from build123d import *

# Parameters (mm, degrees)
SKETCH1_W           = 4.1
SKETCH1_H           = 15
SKETCH1_W_2         = 15
SKETCH1_H_2         = 4.1
BOSS_EXTRUDE1_DEPTH = 4.1


with BuildPart() as part:
    # Sketch1 → Boss-Extrude1 (new body)
    with BuildSketch(Plane(origin=(0, 0, 0), x_dir=(1, 0, 0), z_dir=(0, 1, 0))):
        Polygon((0, 45.9), (0, 0), (22.5, 0), (22.5, 4.1), (37.5, 4.1), (37.5, 0), (60, 0), (60, 45.9), align=None)
        with Locations((7.05, 34.55)):
            Rectangle(SKETCH1_W, SKETCH1_H, mode=Mode.SUBTRACT)
        with Locations((7.05, 15.45)):
            Rectangle(SKETCH1_W, SKETCH1_H, mode=Mode.SUBTRACT)
        with Locations((52.95, 34.55)):
            Rectangle(SKETCH1_W, SKETCH1_H, mode=Mode.SUBTRACT)
        with Locations((52.95, 15.45)):
            Rectangle(SKETCH1_W, SKETCH1_H, mode=Mode.SUBTRACT)
        with Locations((30, 25)):
            Rectangle(SKETCH1_W_2, SKETCH1_H_2, mode=Mode.SUBTRACT)
    extrude(amount=BOSS_EXTRUDE1_DEPTH)


solid = part.part
Can you work these out from the model? Positions are in its coordinate system, mm. A direction names the side the tool comes from. Give positions to 0.01 mm unless a question says otherwise; leave off trailing zeros. Write each loop counter-clockwise with the first axis right and the second up, starting at its lowest first coordinate (ties: lowest second). Pieces come first, ordered by that corner, then holes. Notation, with made-up numbers: (-30.5, -5.5) -> (6.5, -5.5) arc R10 cw to (6.5, 3.5) -> close; hole circle Ø6 at (-31.75, 60.5). An arc over 180 degrees is marked (long way). Answer as a JSON object with one key per item and string values. Group by question number.
Item 1: Suppose I cut it at A-A (z = -34.5). Please give me the cut outline in (x, y), plus the area to 3 significant figures.
Item 2: Suppose I cut it at B-B (x = 32). Please give me the cut outline in (y, z).
Item 3: Please list where these lines run through material, in increasing order: line 1 (X direction, y = 3.8, z = -15); line 2 (Z direction, x = 6.5, y = 0.65); line 3 (X direction, y = 2.6, z = -25.5). Write a range as [from, to].
Item 4: Suppose I cut it at C-C (x = 6). Please give me the cut outline in (y, z).
Item 5: Suppose I cut it at D-D (z = -24.5). Please give me the cut outline in (x, y).
Item 6: For faces 1 (the face through (37.5, 2, -2)), 2 (the face through (7, 2, -42.05)), 3 (the face through (30, 4.1, -28)), which set-ups out of +Z, -Z, +X, -X, +Y, -Y let a thin tool reach every point of the face, with its end or its side?
Item 7: I'm going to push a flat-ended pin straight in: P1, Ø1.2, axis at x = 32.5, y = 1.5, coming from the +Z side. Where does the tip first touch, or does it pass through?
Item 8: We'd pull the mould along X, two halves only. Please class faces 4 (the face through (49, 2, 0)), 5 (the face through (9.1, 2, -15)), 6 (the face through (60, 2, -23)): +X half, -X half, draft (parallel to the pull), parting line (faces both ways), or undercut.
Findings:
{
 "1": {"outline": "(0, 0) -> (5, 0) -> (5, 4.1) -> (0, 4.1) -> close; (9.1, 0) -> (50.9, 0) -> (50.9, 4.1) -> (9.1, 4.1) -> close; (55, 0) -> (60, 0) -> (60, 4.1) -> (55, 4.1) -> close", "area": "212 mm²"},
 "2": {"outline": "(0, -45.9) -> (4.1, -45.9) -> (4.1, -27.05) -> (0, -27.05) -> close; (0, -22.95) -> (4.1, -22.95) -> (4.1, -4.1) -> (0, -4.1) -> close"},
 "3": {"line 1": "x = [0, 5], [9.1, 50.9], [55, 60]", "line 2": "z = [-45.9, -42.05], [-27.05, -22.95], [-7.95, 0]", "line 3": "x = [0, 22.5], [37.5, 60]"},
 "4": {"outline": "(0, -45.9) -> (4.1, -45.9) -> (4.1, -42.05) -> (0, -42.05) -> close; (0, -27.05) -> (4.1, -27.05) -> (4.1, -22.95) -> (0, -22.95) -> close; (0, -7.95) -> (4.1, -7.95) -> (4.1, 0) -> (0, 0) -> close"},
 "5": {"outline": "(0, 0) -> (22.5, 0) -> (22.5, 4.1) -> (0, 4.1) -> close; (37.5, 0) -> (60, 0) -> (60, 4.1) -> (37.5, 4.1) -> close"},
 "6": {"face 1": "+Z, +Y, -Y", "face 2": "+Y, -Y", "face 3": "+Z, -Z, +X, -X, +Y"},
 "7": {"P1": "stops at z = -4.1"},
 "8": {"face 4": "draft", "face 5": "undercut", "face 6": "+X half"}
}
